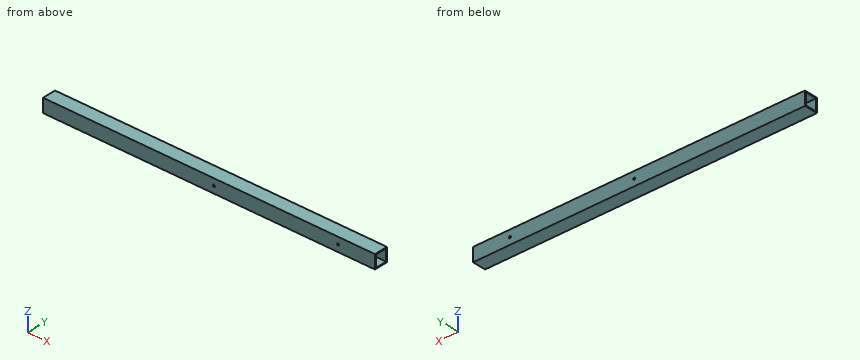
from build123d import *

# Parameters (mm, degrees)
SKETCH1_W                = 1085.85
SKETCH1_H                = 44.45
BOSS_EXTRUDE1_DEPTH      = 44.45
SHELL1_T                 = -3.175
H_0_266_DIAMETER_HOLE1_D = 6.7564


with BuildPart() as part:
    # Sketch1 → Boss-Extrude1 (new body)
    with BuildSketch(Plane.XY):
        with Locations((542.925, 22.225)):
            Rectangle(SKETCH1_W, SKETCH1_H)
    extrude(amount=BOSS_EXTRUDE1_DEPTH)

    # Shell1
    shell1_openings = [part.faces().sort_by_distance(p)[0] for p in [
        (1085.85, 22.225, 22.225),
        (0, 22.225, 22.225),
    ]]
    offset(amount=SHELL1_T, openings=shell1_openings, kind=Kind.INTERSECTION)

    # H (0.266) Diameter Hole1 (through all)
    with Locations(Plane(origin=(0, 44.45, 0), x_dir=(1, 0, 0), z_dir=(0, 1, 0))):
        with Locations((965.2, -22.225), (558.8, -22.225)):
            Hole(H_0_266_DIAMETER_HOLE1_D / 2)


solid = part.part
Work out the finished part from the listing and answer in its coordinate system (mm). Round coordinates to 2 decimals unless told otherwise and drop trailing zeros. Write each loop counter-clockwise with the first axis right and the second up, starting at its lowest first coordinate (ties: lowest second). Pieces come first, ordered by that corner, then holes. Notation, with made-up numbers: (42, 44.25) -> (55, 44.25) arc R26 ccw to (55, 71.25) -> close; hole circle Ø10 at (46.25, -3). An arc over 180 degrees is marked (long way). Answer as CSV lines item,"result". Start each with the question number.
(1) Find the intervals of material crossed by probe 1 along Z at (x, y) = (385, 27) (3 decimals); probe 2 along Z at (x, y) = (558.8, 2.2), in increasing order.
(2) The part is cut by section B-B, the plane x = 417. Give the vertices of the cut face in (y, z) (3 decimals), then the cut area to 3 significant figures.
(3) The part is cut by section A-A, the plane y = 32. Give the vertices of the cut face in (x, z) (3 decimals), then the cut area to 3 significant figures.
(4) This flat-tipped pin is pushed along its axis until it touches: pin 1 (4 mm diameter, centred on x = 558.8, z = 22.225, fed in from +Y). Where does it stop, or does it pass through?
Output values:
1,probe 1,"z = 0 to 3.175, 41.275 to 44.45"
1,probe 2,"z = 0 to 18.85, 25.6 to 44.45"
2,outline,"(0, 0) -> (44.45, 0) -> (44.45, 44.45) -> (0, 44.45) -> close; hole (3.175, 3.175) -> (41.275, 3.175) -> (41.275, 41.275) -> (3.175, 41.275) -> close"
2,area,"524 mm²"
3,outline,"(0, 0) -> (1085.85, 0) -> (1085.85, 3.175) -> (0, 3.175) -> close; (0, 41.275) -> (1085.85, 41.275) -> (1085.85, 44.45) -> (0, 44.45) -> close"
3,area,"6,900 mm²"
4,pin 1,"passes through"
